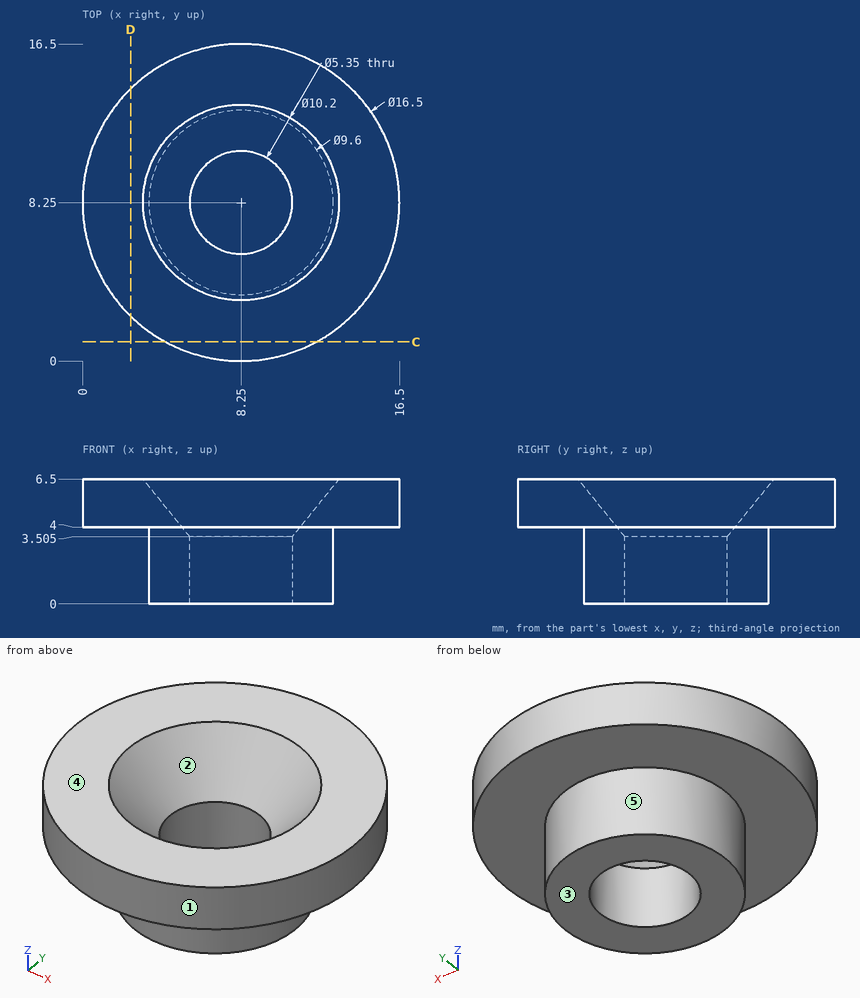
Print and shaded views of the part. All mm, measured from the part's lowest x, y and z. A direction names the side the tool comes from. Coordinates: 2 decimals unless noted, no trailing zeros. Loops run counter-clockwise (first coordinate to the right, second up) from the corner with the lowest first, then second, coordinate; pieces in that order, holes last. Notation, with made-up numbers: (87.25, -38.5) -> (143.25, -38.5) arc R16 cw to (143.25, -7.5) -> close; hole circle Ø4 at (1, -27). An arc over 180 degrees is marked (long way). Use one line per item in the form item = value. Start each with the question number.
(1) Cut at D-D on x = 2.5. Give the cut face in (y, z), and give its area (3 significant figures).
(2) Pull direction Y, two halves, no side cores. Call the marked faces 1, 2 and 3: pulls with the +Y half, pulls with the -Y half, needs draft (parallel to the pull), parting line crosses it, or undercut.
(3) Cut at C-C on y = 1. Give the cut face in (x, z).
(4) Probe probe 1 along Z at (x, y) = (1.5, 4); probe 2 along X at (y, z) = (7.5, 1); probe 3 along Y at (x, z) = (5, 0.5). List the from-to ranges inside material, lowest first. Write a range as from..to.
(5) Flat gauge pins, fed straight in: pin 1 (6 mm diameter, centred on x = 8.25, y = 8.25, fed in from +Z) (1 decimal); pin 2 (2 mm diameter, centred on y = 13, z = 5, fed in from -X); pin 3 (1.5 mm diameter, centred on y = 12, z = 5.5, fed in from -X) (1 decimal). Where does each tip first touch, or does it go through?
(6) Tool access for the marked faces 4 and 5: list every direction of +Z, -Z, +X, -X, +Y, -Y with a clear straight run to the whole face (end or side of a thin tool).
Values:
q1.outline = (2.33, 4) -> (14.17, 4) -> (14.17, 6.5) -> (2.33, 6.5) -> close
q1.area = 29.6 mm2
q2.face_1 = parting line crosses it
q2.face_2 = undercut
q2.face_3 = needs draft
q3.outline = (4.31, 4) -> (12.19, 4) -> (12.19, 6.5) -> (4.31, 6.5) -> close
q4.probe_1 = 4..6.5
q4.probe_2 = 3.51..5.68, 10.82..12.99
q4.probe_3 = 4.72..11.78
q5.pin_1 = 3.9
q5.pin_2 = 0.9
q5.pin_3 = 0.6
q6.face_4 = +Z, +X, -X, +Y, -Y
q6.face_5 = -Z
